from build123d import *

# Parameters (mm, degrees)
P_IDAT_VYSUNUT_M1_DEPTH  = 2
SKICA2_W                 = 20
SKICA2_H                 = 2
P_IDAT_VYSUNUT_M2_DEPTH  = 15
SKICA3_W                 = 5.5
SKICA3_H                 = 3
ODEBRAT_VYSUNUT_M1_DEPTH = 15
SKICA5_W                 = 20
SKICA5_H                 = 15
SKICA5_W_2               = 5.5
SKICA5_H_2               = 3
P_IDAT_VYSUNUT_M3_DEPTH  = 3


with BuildPart() as part:
    # Skica1 → Přidat vysunutím1 (new body)
    with BuildSketch(Plane.XY):
        Polygon((0, 0), (5, 0), (5, -2), (10, -2), (10, 4.082474227), (10, 13), (30, 13), (30, -2), (35, -2), (35, 18), (5, 18), (5, 5), (0, 5), align=None)
    extrude(amount=P_IDAT_VYSUNUT_M1_DEPTH)

    # Skica2 → Přidat vysunutím2 (add)
    with BuildSketch(Plane(origin=(0, 18, 0), x_dir=(1, 0, 0), z_dir=(0, 1, 0))):
        with Locations((20, -1)):
            Rectangle(SKICA2_W, SKICA2_H)
    extrude(amount=P_IDAT_VYSUNUT_M2_DEPTH)

    # Skica3 → Odebrat vysunutím1 (cut)
    with BuildSketch(Plane.XY.offset(2)):
        with Locations((20, 28)):
            Rectangle(SKICA3_W, SKICA3_H)
    extrude(amount=-ODEBRAT_VYSUNUT_M1_DEPTH, mode=Mode.SUBTRACT)

    # Skica5 → Přidat vysunutím3 (add)
    with BuildSketch(Plane.XY.offset(2)):
        with Locations((20, 25.5)):
            Rectangle(SKICA5_W, SKICA5_H)
        with Locations((20, 28)):
            Rectangle(SKICA5_W_2, SKICA5_H_2, mode=Mode.SUBTRACT)
    extrude(amount=P_IDAT_VYSUNUT_M3_DEPTH)


solid = part.part
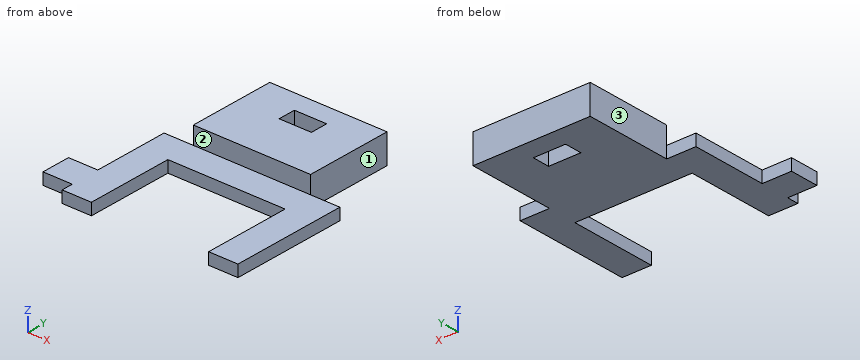
Build history of the part. All positions in model axes, mm. Face numbers are marked on the shaded views. A direction names the side the tool comes from. Give positions to 0.01 mm unless a question says otherwise; leave off trailing zeros. Order: outer loops, then holes, each group sorted by start corner. A loop starts at its lowest first (then second) coordinate and runs counter-clockwise, first axis right, second up. Notation, with made-up numbers: M 25.5,-38 L 79.5,-38 A10 cw 79.5,-26 Z; hole C 48.5,16.25 d1. An arc over 180 degrees is marked long. Use one line per item in the form item = value.
1) Saw through at B-B (x = 20). Give the cut face in (y, z), plus the area to 3 significant figures.
Calculated:
outline = M 13,0 L 26.5,0 L 26.5,5 L 18,5 L 18,2 L 13,2 Z; M 29.5,0 L 33,0 L 33,5 L 29.5,5 Z
area = 70.0 mm2
2) Saw through at D-D (y = 28). Give the cut face in (x, z), plus the area to 3 significant figures.
Calculated:
outline = M 10,0 L 17.25,0 L 17.25,5 L 10,5 Z; M 22.75,0 L 30,0 L 30,5 L 22.75,5 Z
area = 72.5 mm2
3) Drop flat-ended pins along their axis: pin 1 (1.6 mm diameter, centred on x = 21.5, z = 0.5, fed in from -Y); pin 2 (1.6 mm diameter, centred on x = 3.5, z = 0.5, fed in from -Y); pin 3 (2 mm diameter, centred on x = 6.5, z = 0.5, fed in from +Y); pin 4 (3 mm diameter, centred on x = 12.5, y = 7, fed in from +Z). Give the stop position or say it passes through.
Calculated:
pin_1 = 13
pin_2 = 0
pin_3 = 18
pin_4 = through
4) Probe probe 1 along Y at (x, z) = (18, 0.9); probe 2 along X at (y, z) = (11, 1.95); probe 3 along X at (y, z) = (2, 1.95). List the from-to ranges inside material, lowest first.
Calculated:
probe_1 = 13 to 26.5, 29.5 to 33
probe_2 = 5 to 10, 30 to 35
probe_3 = 0 to 10, 30 to 35
5) Saw through at A-A (y = 4). Give the cut face in (x, z).
Calculated:
outline = M 0,0 L 10,0 L 10,2 L 0,2 Z; M 30,0 L 35,0 L 35,2 L 30,2 Z
6) Tool access for the marked faces 1, 2 and 3: list every direction of +Z, -Z, +X, -X, +Y, -Y with a clear straight run to the whole face (end or side of a thin tool).
Calculated:
face_1 = +Z, -Z, +X, +Y
face_2 = +Z, +X, -X, -Y
face_3 = +Z, -Z, -X, +Y
7) Saw through at C-C (z = 3.7). Give the cut face in (x, y).
Calculated:
outline = M 10,18 L 30,18 L 30,33 L 10,33 Z; hole M 17.25,26.5 L 22.75,26.5 L 22.75,29.5 L 17.25,29.5 Z
